from build123d import *

# Parameters (mm, degrees)
SKETCH2_R           = 1.5
BOSS_EXTRUDE1_DEPTH = 2


with BuildPart() as part:
    # Sketch2 → Boss-Extrude1 (new body)
    with BuildSketch(Plane(origin=(0, 0, 0), x_dir=(0, 0, -1), z_dir=(1, 0, 0))):
        with BuildLine():
            Line((390.798820845, 95), (275.798820845, 95))
            ThreePointArc((275.798820845, 95), (268.727753033, 92.071067812), (265.798820845, 85))
            Line((265.798820845, 85), (265.798820845, 10))
            ThreePointArc((265.798820845, 10), (268.727753033, 2.928932188), (275.798820845, 0))
            Line((275.798820845, 0), (357.798820845, 0))
            ThreePointArc((357.798820845, 0), (361.334354751, 1.464466094), (362.798820845, 5))
            Line((362.798820845, 5), (362.798820845, 25))
            ThreePointArc((362.798820845, 25), (365.727753033, 32.071067812), (372.798820845, 35))
            Line((372.798820845, 35), (395.798820845, 35))
            ThreePointArc((395.798820845, 35), (399.334354751, 36.464466094), (400.798820845, 40))
            Line((400.798820845, 40), (400.798820845, 85))
            ThreePointArc((400.798820845, 85), (397.869888657, 92.071067812), (390.798820845, 95))
        make_face()
        with Locations((371.798820845, 86.5)):
            Circle(SKETCH2_R, mode=Mode.SUBTRACT)
        with Locations((391.798820845, 86.5)):
            Circle(SKETCH2_R, mode=Mode.SUBTRACT)
        with Locations((391.798820845, 40.9)):
            Circle(SKETCH2_R, mode=Mode.SUBTRACT)
        with Locations((371.798820845, 40.9)):
            Circle(SKETCH2_R, mode=Mode.SUBTRACT)
        with Locations((356.298820845, 7)):
            Circle(SKETCH2_R, mode=Mode.SUBTRACT)
        with Locations((274.798820845, 7)):
            Circle(SKETCH2_R, mode=Mode.SUBTRACT)
        with Locations((274.798820845, 86.5)):
            Circle(SKETCH2_R, mode=Mode.SUBTRACT)
        with Locations((356.298820845, 86.5)):
            Circle(SKETCH2_R, mode=Mode.SUBTRACT)
        with BuildLine():
            Line((284.798820845, 42), (346.298820845, 42))
            Line((346.298820845, 42), (346.298820845, 27))
            ThreePointArc((346.298820845, 27), (343.369888657, 19.928932188), (336.298820845, 17))
            Line((336.298820845, 17), (294.798820845, 17))
            ThreePointArc((294.798820845, 17), (287.727753033, 19.928932188), (284.798820845, 27))
            Line((284.798820845, 27), (284.798820845, 42))
        make_face(mode=Mode.SUBTRACT)
        with BuildLine():
            Line((336.298820845, 76.5), (294.798820845, 76.5))
            ThreePointArc((294.798820845, 76.5), (287.727753033, 73.571067812), (284.798820845, 66.5))
            Line((284.798820845, 66.5), (284.798820845, 51.5))
            Line((284.798820845, 51.5), (346.298820845, 51.5))
            Line((346.298820845, 51.5), (346.298820845, 66.5))
            ThreePointArc((346.298820845, 66.5), (343.369888657, 73.571067812), (336.298820845, 76.5))
        make_face(mode=Mode.SUBTRACT)
        with BuildLine():
            Line((383.798820845, 77), (379.798820845, 77))
            ThreePointArc((379.798820845, 77), (377.677500501, 76.121320344), (376.798820845, 74))
            Line((376.798820845, 74), (376.798820845, 51.9))
            ThreePointArc((376.798820845, 51.9), (377.677500501, 49.778679656), (379.798820845, 48.9))
            Line((379.798820845, 48.9), (383.798820845, 48.9))
            ThreePointArc((383.798820845, 48.9), (385.920141188, 49.778679656), (386.798820845, 51.9))
            Line((386.798820845, 51.9), (386.798820845, 74))
            ThreePointArc((386.798820845, 74), (385.920141188, 76.121320344), (383.798820845, 77))
        make_face(mode=Mode.SUBTRACT)
    extrude(amount=BOSS_EXTRUDE1_DEPTH)


solid = part.part
Geometry: final body of the model. Coordinates: model frame, mm. A direction names the side the tool comes from. Give positions to 0.01 mm unless a question says otherwise; leave off trailing zeros. Order: outer loops, then holes, each group sorted by start corner. A loop starts at its lowest first (then second) coordinate and runs counter-clockwise, first axis right, second up. Notation, with made-up numbers: (4.25, 15) -> (39.25, 15) arc R28 ccw to (39.25, 44) -> close; hole circle Ø5 at (47.5, 48). An arc over 180 degrees is marked (long way). Answer as a JSON object with one key per item and string values.
Q1. Access query for faces 5 (the cylindrical face through (0.99, 73.65, -287.81)), 6 (the cylindrical face through (0.99, 91.99, -397.95)). Directions: +Z, -Z, +X, -X, +Y, -Y. A direction counts if a zero-diameter tool reaches every point of the face in a straight line with its end or side. Return the directions, or none.
Entries:
{"face 5": "+X, -X", "face 6": "-Z, +X, -X, +Y"}
Q2. Material intervals for probe 1 along Z at (x, y) = (1.6, 54); probe 2 along Y at (x, z) = (1.65, -311.5); probe 3 along Y at (x, z) = (0.55, -379.5), sorted ascending.
Entries:
{"probe 1": "z = -400.8 to -386.8, -376.8 to -346.3, -284.8 to -265.8", "probe 2": "y = 0 to 17, 42 to 51.5, 76.5 to 95", "probe 3": "y = 35 to 48.91, 76.99 to 95"}
Q3. Section A-A (y = 61). Output: boundary loops of the cut face in (x, z).
Entries:
{"outline": "(0, -400.8) -> (2, -400.8) -> (2, -386.8) -> (0, -386.8) -> close; (0, -376.8) -> (2, -376.8) -> (2, -346.3) -> (0, -346.3) -> close; (0, -284.8) -> (2, -284.8) -> (2, -265.8) -> (0, -265.8) -> close"}
Q4. Draft query along Z for faces 1 (the cylindrical face through (0.99, 92.15, -268.81)), 2 (the cylindrical face through (0.99, 41.35, -393.23)), 3 (the cylindrical face through (0.99, 19.85, -287.81)), 4 (the flat face through (0, 48, -332)). Return one class per face: released by +Z, released by -Z, zero draft, split by the parting line, or undercut.
Entries:
{"face 1": "released by +Z", "face 2": "undercut", "face 3": "undercut", "face 4": "zero draft"}
Q5. First-contact query: pin 1 (0.6 mm diameter, centred on x = 0.5, y = 18.5, fed in from -Z); pin 2 (2 mm diameter, centred on y = 53, z = -342, fed in from -X). Flat tips, straight axial feed; report the tip coordinate or a pass-through.
Entries:
{"pin 1": "stops at z = -362.8", "pin 2": "passes through"}
Q6. Section C-C (y = 86.5). Output: boundary loops of the cut face in (x, z), plus the area to 3 significant figures.
Entries:
{"outline": "(0, -400.69) -> (2, -400.69) -> (2, -393.3) -> (0, -393.3) -> close; (0, -390.3) -> (2, -390.3) -> (2, -373.3) -> (0, -373.3) -> close; (0, -370.3) -> (2, -370.3) -> (2, -357.8) -> (0, -357.8) -> close; (0, -354.8) -> (2, -354.8) -> (2, -276.3) -> (0, -276.3) -> close; (0, -273.3) -> (2, -273.3) -> (2, -265.91) -> (0, -265.91) -> close", "area": "246 mm^2"}
Q7. Section B-B (z = -297.5). Output: boundary loops of the cut face in (x, y).
Entries:
{"outline": "(0, 0) -> (2, 0) -> (2, 17) -> (0, 17) -> close; (0, 42) -> (2, 42) -> (2, 51.5) -> (0, 51.5) -> close; (0, 76.5) -> (2, 76.5) -> (2, 95) -> (0, 95) -> close"}
Q8. Section D-D (x = 1.25). State how many separate pieces and enclosed holes the cut face has, plus the area to 3 significant figures.
Entries:
{"separate pieces": "1", "enclosed holes": "11", "area": "8,120 mm^2"}
